For this review, take the finished solid that the model builds, in its own axes (mm). Round coordinates to 2 decimals unless told otherwise and drop trailing zeros. Answer in a Markdown table with one row per item. Add a question column.
```python
from build123d import *

# Parameters (mm, degrees)
F0_R     = 3
F1_DEPTH = 350


with BuildPart() as f1:
    # F0 (on Top) → F1 (new body)
    with BuildSketch(Plane.XY):
        Polygon((-12, 10), (-20, 10), (-20, 2), (-17, 2), (-17, -2), (-20, -2), (-20, -10), (-12, -10), (-12, -7), (-8, -7), (-8, -10), (8, -10), (8, -7), (12, -7), (12, -10), (20, -10), (20, -2), (17, -2), (17, 2), (20, 2), (20, 10), (12, 10), (12, 7), (8, 7), (8, 10), (-8, 10), (-8, 7), (-12, 7), align=None)
        with Locations((-10, 0)):
            Circle(F0_R, mode=Mode.SUBTRACT)
        with Locations((10, 0)):
            Circle(F0_R, mode=Mode.SUBTRACT)
    extrude(amount=F1_DEPTH)


solid = f1.part
```
1. Clearance check with flat-ended pins moving along their axes: pin 1 Ø2 at (x, z) = (-10.5, 132) entering from -Y; pin 2 Ø5 at (x, y) = (-10, 0) entering from +Z; pin 3 Ø1.2 at (y, z) = (0.5, 167) entering from +X. State where each tip first meets the part, or that it passes through.
2. Consider section A-A on z = 52. State how many separate pieces and enclosed holes the cut face has, plus the area to 3 significant figures.
3. To check wall thickness, follow probe 1 along X at (y, z) = (2.25, 66); probe 2 along X at (y, z) = (-0.25, 224); probe 3 along Y at (x, z) = (10, 190). State the ranges of each line that lie inside material, in increasing order. Write a range as [from, to].
4. The part is to be moulded in two halves that separate along Y. For faces 1 (the cylindrical face through (-12.4, -1.8, 172.6)), 2 (the flat face through (-20, 6, 173)), 3 (the flat face through (16, 10, 173)), 4 (the flat face through (16, -10, 173)), say which applies: pulls with the +Y half, pulls with the -Y half, needs draft (parallel to the pull), parting line crosses it, or undercut.
Solved:
| question | item | result |
|---|---|---|
| 1 | pin 1 | stops at y = -7 |
| 1 | pin 2 | passes through |
| 1 | pin 3 | stops at x = 17 |
| 2 | separate pieces | 1 |
| 2 | enclosed holes | 2 |
| 2 | area | 671 mm^2 |
| 3 | probe 1 | x = [-20, -11.98], [-8.02, 8.02], [11.98, 20] |
| 3 | probe 2 | x = [-17, -12.99], [-7.01, 7.01], [12.99, 17] |
| 3 | probe 3 | y = [-7, -3], [3, 7] |
| 4 | face 1 | undercut |
| 4 | face 2 | needs draft |
| 4 | face 3 | pulls with the +Y half |
| 4 | face 4 | pulls with the -Y half |
